Check sheet for the modelled part. Datum: model origin and axes. Units: mm. Face numbers are marked on the shaded views. A direction names the side the tool comes from. Round coordinates to 2 decimals unless told otherwise and drop trailing zeros. Loops run counter-clockwise (first coordinate to the right, second up) from the corner with the lowest first, then second, coordinate; pieces in that order, holes last. Notation, with made-up numbers: (7.5, -31.75) - (42.5, -31.75) arc R11 ccw to (42.5, -16.75) - close; hole circle Ø2 at (28.25, 4). An arc over 180 degrees is marked (long way). Put each result on its own line as item: value. Start each with the question number.
Autodesk Inventor part; units mm, degrees
ref_plane "Arbeitsebene1" through (0, 0, 0) normal (0, 1, 0) x (-1, 0, 0)
ref_plane "YZ Plane" through (0, 0, 0) normal (1, 0, 0) x (0, 1, 0)
ref_plane "XY Plane" through (0, 0, 0) normal (0, 0, 1) x (1, 0, 0)
sketch "Skizze1" plane through (0, 0, 0) normal (0, 1, 0) x (-1, 0, 0)
  line L0 (0, 0) -> (18, 0)
  line L1 (18, 0) -> (18, -6)
  arc A0 (18, -6) -> (20, -8) centre (20, -6) ccw
  line L2 (20, -8) -> (20, -13)
  line L3 (20, -13) -> (0, -13)
  line L4 (0, -13) -> (0, 0)
  dimension "d0" = 5
  dimension "d2" = 40
  dimension "d3" = 36
  dimension "d12" = 13
revolve "Umdrehung1" add sketch "Skizze1" angle 360 about axis through (0, 0, -13) along (0, 0, 1)
ref_plane "Arbeitsebene1" through (0, 0, 0) normal (0, 1, 0) x (-1, 0, 0)
sketch "Skizze2" plane through (0, 0, 0) normal (0, 1, 0) x (-1, 0, 0)
  line L0 (18, 0) -> (-18, 0)
  line L1 (20, -13) -> (-20, -13)
  line L2 (5.75, 0) -> (3.3056, -11.5)
  line L3 (3.3056, -11.5) -> (10, -11.5)
  line L4 (10, -11.5) -> (10, -12.0712)
  line L5 (10, -12.0712) -> (10, -12.0712)
  line L6 (10, -12.0712) -> (10, -13)
  line L7 (0, 0) -> (0, -13)
  line L8 (5.75, 0) -> (0, 0)
  dimension "d6" = 1.5
  dimension "d7" = 12
  dimension "d8" = 11.5
  dimension "d9" = 20
revolve "Umdrehung2" cut sketch "Skizze2" angle 360 about axis through (0, 0, 0) along (0, 0, -1)
properties part number "Mitnehmer" material "Lead"
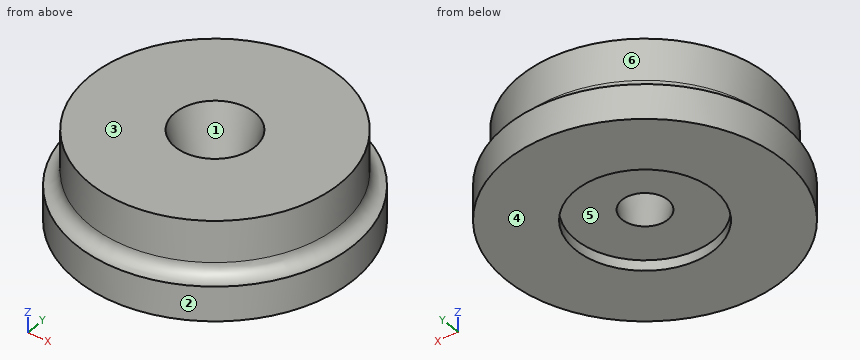
Q1. Cross-section at A-A on x = 0. Enter the section's corners in (y, z), and give its area (3 significant figures).
Q2. Draft check along X on the marked faces 1, 2 and 3. Enter one of: +X half, -X half, draft (parallel to the pull), parting line (faces both ways), or undercut.
Q3. Material ranges on line 1 (Y direction, x = 0, z = -11.8); line 2 (Z direction, x = 8.5, y = -4.5); line 3 (X direction, y = 2.5, z = -9.5), recorded low to high. Write a range as from..to.
Q4. Depth check by flat-ended pin: pin 1 Ø6 at (x, z) = (13.5, -11) entering from -Y; pin 2 Ø3 at (y, z) = (-11, -9) entering from +X; pin 3 Ø16 at (x, y) = (0, 0) entering from -Z. Enter the tip coordinate at first touch or a pass-through.
Q5. Set-up check for the marked faces 4, 5 and 6: record each of +Z, -Z, +X, -X, +Y, -Y from which the full face is reachable in a straight line by a thin tool's end or side.
Answer list:
1. outline: (-20, -13) - (-10, -13) - (-10, -11.5) - (-3.31, -11.5) - (-5.75, 0) - (-18, 0) - (-18, -6) arc R2 cw to (-20, -8) - close; (3.31, -11.5) - (10, -11.5) - (10, -13) - (20, -13) - (20, -8) arc R2 cw to (18, -6) - (18, 0) - (5.75, 0) - close
1. area: 356 mm2
2. face 1: undercut
2. face 2: parting line
2. face 3: draft
3. line 1: y = -20..-10, 10..20
3. line 2: z = -11.5..0
3. line 3: x = -19.84..-2.77, 2.77..19.84
4. pin 1: stops at y = -17.02
4. pin 2: stops at x = 17.6
4. pin 3: stops at z = -11.5
5. face 4: -Z, +X, -X, +Y, -Y
5. face 5: -Z
5. face 6: +Z
